```python
from build123d import *

# Parameters (mm, degrees)
CROQUIS1_W              = 30
CROQUIS1_H              = 30
SALIENTE_EXTRUIR2_DEPTH = 3
SALIENTE_EXTRUIR3_DEPTH = 50
CROQUIS3_R              = 2
SALIENTE_EXTRUIR4_DEPTH = 52.5


with BuildPart() as part:
    # Croquis1 → Saliente-Extruir2 (new body)
    with BuildSketch(Plane(origin=(0, 0, 0), x_dir=(1, 0, 0), z_dir=(0, 1, 0))):
        Rectangle(CROQUIS1_W, CROQUIS1_H)
    extrude(amount=-SALIENTE_EXTRUIR2_DEPTH)

    # Croquis2 → Saliente-Extruir3 (add)
    with BuildSketch(Plane.XZ.offset(3)):
        Polygon((-15, 15), (-12, 15), (-12, -12), (12, -12), (12, 15), (15, 15), (15, -15), (12, -15), (-12, -15), (-15, -15), align=None)
    extrude(amount=SALIENTE_EXTRUIR3_DEPTH)

    # Croquis3 → Saliente-Extruir4 (add)
    with BuildSketch(Plane.XZ.offset(3)):
        with Locations(Location((-7, 0, 0), (0, 0, 90))):
            Circle(CROQUIS3_R)
        with Locations(Location((7, 0, 0), (0, 0, 90))):
            Circle(CROQUIS3_R)
    extrude(amount=SALIENTE_EXTRUIR4_DEPTH)


solid = part.part
```
Model file for the job. Use its own axes, mm. A direction names the side the tool comes from. Give positions to 0.01 mm unless a question says otherwise; leave off trailing zeros. Loops run counter-clockwise (first coordinate to the right, second up) from the corner with the lowest first, then second, coordinate; pieces in that order, holes last. Notation, with made-up numbers: (-30.5, 44.25) -> (-1.5, 44.25) arc R15 ccw to (-1.5, 64.25) -> close; hole circle Ø3 at (0.25, 45.25). An arc over 180 degrees is marked (long way). Write each question's results on one line, items separated by ' | '.
(1) Flat gauge pin, fed straight in: pin 1 Ø1 at (x, z) = (2.5, 11) entering from -Y. Where does the tip first touch, or does it go through?
Geometry results:
pin 1: stops at y = -3
(2) Cut at C-C on z = 0. List the corners of the cut face in (x, y), and give its area (3 significant figures).
Geometry results:
outline: (-15, -53) -> (-12, -53) -> (-12, -3) -> (-9, -3) -> (-9, -55.5) -> (-5, -55.5) -> (-5, -3) -> (5, -3) -> (5, -55.5) -> (9, -55.5) -> (9, -3) -> (12, -3) -> (12, -53) -> (15, -53) -> (15, 0) -> (-15, 0) -> close | area: 810 mm²
(3) Tool access for faces 4 (the flat face through (0, -26, -15)), 5 (the flat face through (-12, -28, 2)), 6 (the flat face through (0, -28, -12)): list every direction of +Z, -Z, +X, -X, +Y, -Y with a clear straight run to the whole face (end or side of a thin tool).
Geometry results:
face 4: -Z, +X, -X, +Y, -Y | face 5: +Z, -Y | face 6: -Y
(4) Cut at D-D on x = 7. List the corners of the cut face in (y, z).
Geometry results:
outline: (-55.5, -2) -> (-3, -2) -> (-3, -12) -> (-53, -12) -> (-53, -15) -> (0, -15) -> (0, 15) -> (-3, 15) -> (-3, 2) -> (-55.5, 2) -> close
(5) Cut at B-B on x = 1.75. List the corners of the cut face in (y, z).
Geometry results:
outline: (-53, -15) -> (0, -15) -> (0, 15) -> (-3, 15) -> (-3, -12) -> (-53, -12) -> close
(6) Cut at A-A on y = -39. List the corners of the cut face in (x, z), and give its area (3 significant figures).
Geometry results:
outline: (-15, -15) -> (15, -15) -> (15, 15) -> (12, 15) -> (12, -12) -> (-12, -12) -> (-12, 15) -> (-15, 15) -> close; circle Ø4 at (-7, 0); circle Ø4 at (7, 0) | area: 277 mm²
(7) Probe line 1 along X through (y, z) = (-22, 0); line 2 along X through (y, z) = (-34.5, -7.5); line 3 along X through (y, z) = (-38.5, 1.75). List the from-to ranges inside material, lowest first.
Geometry results:
line 1: x = -15 to -12, -9 to -5, 5 to 9, 12 to 15 | line 2: x = -15 to -12, 12 to 15 | line 3: x = -15 to -12, -7.97 to -6.03, 6.03 to 7.97, 12 to 15
(8) Pull direction Z, two halves, no side cores. Call faces 1 (the cylindrical face through (7, -29, -2)), 2 (the flat face through (-12.3, -20.5, 15)), 3 (the flat face through (7, -55.5, 0)): released by +Z, released by -Z, zero draft, split by the parting line, or undercut.
Geometry results:
face 1: undercut | face 2: released by +Z | face 3: zero draft
